CAD build for the part. Positions are in the model's coordinates, mm. Give positions to 0.01 mm unless a question says otherwise; leave off trailing zeros. Order: outer loops, then holes, each group sorted by start corner. A loop starts at its lowest first (then second) coordinate and runs counter-clockwise, first axis right, second up. Notation, with made-up numbers: (31.25, -31) -> (46.25, -31) arc R29 ccw to (46.25, -8) -> close; hole circle Ø8 at (89, -10). An arc over 180 degrees is marked (long way). Use one line per item in the form item = value. Start each with the question number.
1) Cut at B-B, the plane z = 1.25. Give the cut face in (x, y), and give its area (3 significant figures).
2) Cut at C-C, the plane y = 5.75. Give the cut face in (x, z).
3) Drop flat-ended pins along their axis: P1, Ø0.6, axis at x = 22, z = 0, coming from the -Y side; P2, Ø0.9, axis at x = -9, y = 10.5, coming from the -Z side. Give the stop position or say it passes through.
4) Probe line 1 (Y direction, x = 28, z = 0); line 2 (X direction, y = 4, z = 0). List the from-to ranges inside material, lowest first.
5) Cut at A-A, the plane x = 21. Give the cut face in (y, z).
from build123d import *

# Parameters (mm, degrees)
SKETCH_1_R      = 0.4
EXTRUDE_1_DEPTH = 10
SKETCH_2_W      = 80
SKETCH_2_H      = 0.8
EXTRUDE_2_DEPTH = 0.8
FILLET_1_R      = 0.4
SKETCH_3_R      = 0.4
EXTRUDE_3_DEPTH = 3.4
SKETCH_4_R      = 0.4
EXTRUDE_4_DEPTH = 3.4


with BuildPart() as part:
    # 草图1 → 凸台-拉伸1 (new body)
    with BuildSketch(Plane(origin=(0, 0, 0), x_dir=(1, 0, 0), z_dir=(0, 1, 0))):
        with Locations(Location((0, 0, 0), (0, 0, 270))):
            Circle(SKETCH_1_R)
    extrude(amount=EXTRUDE_1_DEPTH)

    # 草图2 → 凸台-拉伸2 (add)
    with BuildSketch(Plane(origin=(0, 10, 0), x_dir=(1, 0, 0), z_dir=(0, 1, 0))):
        Rectangle(SKETCH_2_W, SKETCH_2_H)
    extrude(amount=EXTRUDE_2_DEPTH)

    # 圆角1
    fillet_1_edges = [part.edges().sort_by_distance(p)[0] for p in [
        (40, 10, 0),
        (40, 10.8, 0),
        (-40, 10, 0),
        (-40, 10.8, 0),
    ]]
    fillet(fillet_1_edges, radius=FILLET_1_R - 0.0001)  # a hair under: the kernel refuses the full size

    # 草图3 → 凸台-拉伸3 (add)
    with BuildSketch(Plane.XY.offset(0.4)):
        with Locations((39.6, 10.4)):
            Circle(SKETCH_3_R)
    extrude(amount=EXTRUDE_3_DEPTH)

    # 草图4 → 凸台-拉伸4 (add)
    with BuildSketch(Plane(origin=(0, 0, -0.4), x_dir=(-1, 0, 0), z_dir=(0, 0, -1))):
        with Locations((39.6, 10.4)):
            Circle(SKETCH_4_R)
    extrude(amount=EXTRUDE_4_DEPTH)

    # 草图5 → 旋转1 (revolve)
    with BuildSketch(Plane(origin=(0, 10.4, 0), x_dir=(1, 0, 0), z_dir=(0, 1, 0))):
        Polygon((39.6, -3.8), (39.6, -5.4), (40, -3.8), align=None)
    revolve(axis=Axis((39.6, 10.4, 3.8), (0, 0, 1)))

    # 草图6 → 旋转2 (revolve)
    with BuildSketch(Plane(origin=(0, 10.4, 0), x_dir=(1, 0, 0), z_dir=(0, 1, 0))):
        Polygon((-39.6, 3.8), (-39.6, 5.4), (-40, 3.8), align=None)
    revolve(axis=Axis((-39.6, 10.4, -3.8), (0, 0, -1)))


solid = part.part
Result:
q1.outline = circle Ø0.8 at (39.6, 10.4)
q1.area = 0.503 mm²
q2.outline = circle Ø0.8 at (0, 0)
q3.P1 = 10
q3.P2 = -0.4
q4.line_1 = 10 to 10.8
q4.line_2 = -0.4 to 0.4
q5.outline = (10, -0.4) -> (10.8, -0.4) -> (10.8, 0.4) -> (10, 0.4) -> close
